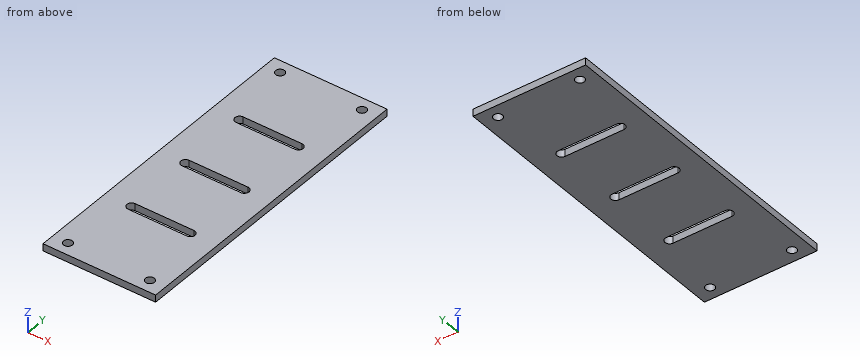
from build123d import *

# Parameters (mm, degrees)
PACK_ACCESS_WITH_STRAP_VENTILATION_PROFI_W = 44
PACK_ACCESS_WITH_STRAP_VENTILATION_PROFI_H = 120
PACK_ACCESS_WITH_STRAP_VENTILATION_PROFI_R = 1.75
PACK_ACCESS_WITH_STRAP_VENTILATION_DEPTH   = 2.8


with BuildPart() as part:
    # Pack access with strap ventilation profile → Pack access with strap ventilation (new body)
    with BuildSketch(Plane.XY):
        Rectangle(PACK_ACCESS_WITH_STRAP_VENTILATION_PROFI_W, PACK_ACCESS_WITH_STRAP_VENTILATION_PROFI_H)
        with Locations((-16, -55)):
            Circle(PACK_ACCESS_WITH_STRAP_VENTILATION_PROFI_R, mode=Mode.SUBTRACT)
        with Locations((-16, 55)):
            Circle(PACK_ACCESS_WITH_STRAP_VENTILATION_PROFI_R, mode=Mode.SUBTRACT)
        with Locations((16, -55)):
            Circle(PACK_ACCESS_WITH_STRAP_VENTILATION_PROFI_R, mode=Mode.SUBTRACT)
        with Locations((16, 55)):
            Circle(PACK_ACCESS_WITH_STRAP_VENTILATION_PROFI_R, mode=Mode.SUBTRACT)
        with BuildLine():
            Line((-11.5, -29.8), (11.5, -29.8))
            ThreePointArc((11.5, -29.8), (13.3, -28), (11.5, -26.2))
            Line((11.5, -26.2), (-11.5, -26.2))
            ThreePointArc((-11.5, -26.2), (-13.3, -28), (-11.5, -29.8))
        make_face(mode=Mode.SUBTRACT)
        with BuildLine():
            Line((-11.5, -1.8), (11.5, -1.8))
            ThreePointArc((11.5, -1.8), (13.3, 0), (11.5, 1.8))
            Line((11.5, 1.8), (-11.5, 1.8))
            ThreePointArc((-11.5, 1.8), (-13.3, 0), (-11.5, -1.8))
        make_face(mode=Mode.SUBTRACT)
        with BuildLine():
            Line((-11.5, 26.2), (11.5, 26.2))
            ThreePointArc((11.5, 26.2), (13.3, 28), (11.5, 29.8))
            Line((11.5, 29.8), (-11.5, 29.8))
            ThreePointArc((-11.5, 29.8), (-13.3, 28), (-11.5, 26.2))
        make_face(mode=Mode.SUBTRACT)
    extrude(amount=PACK_ACCESS_WITH_STRAP_VENTILATION_DEPTH)


solid = part.part
Can you work these out from the model? Positions are in its coordinate system, mm. Coordinates: 2 decimals unless noted, no trailing zeros. Order: outer loops, then holes, each group sorted by start corner. A loop starts at its lowest first (then second) coordinate and runs counter-clockwise, first axis right, second up. Notation, with made-up numbers: M 69.25,65.5 L 75.25,65.5 A5 ccw 75.25,74.5 Z; hole C 21,77 d10. An arc over 180 degrees is marked long. Answer as CSV lines item,"result".
(1) Suppose I cut it at A-A on y = 55. Please give me the cut outline in (x, z), plus the area to 3 significant figures.
Geometry check:
outline,"M -22,0 L -17.75,0 L -17.75,2.8 L -22,2.8 Z; M -14.25,0 L 14.25,0 L 14.25,2.8 L -14.25,2.8 Z; M 17.75,0 L 22,0 L 22,2.8 L 17.75,2.8 Z"
area,"104 mm^2"
(2) Suppose I cut it at D-D on x = 16. Please give me the cut outline in (y, z), plus the area to 3 significant figures.
Geometry check:
outline,"M -60,0 L -56.75,0 L -56.75,2.8 L -60,2.8 Z; M -53.25,0 L 53.25,0 L 53.25,2.8 L -53.25,2.8 Z; M 56.75,0 L 60,0 L 60,2.8 L 56.75,2.8 Z"
area,"316 mm^2"
(3) Suppose I cut it at C-C on y = -28. Please give me the cut outline in (x, z).
Geometry check:
outline,"M -22,0 L -13.3,0 L -13.3,2.8 L -22,2.8 Z; M 13.3,0 L 22,0 L 22,2.8 L 13.3,2.8 Z"
(4) Suppose I cut it at B-B on z = 0.7. Please give me the cut outline in (x, y), plus the area to 3 significant figures.
Geometry check:
outline,"M -22,-60 L 22,-60 L 22,60 L -22,60 Z; hole C -16,-55 d3.5; hole C -16,55 d3.5; hole M -11.5,-29.8 L 11.5,-29.8 A1.8 ccw 11.5,-26.2 L -11.5,-26.2 A1.8 ccw Z; hole M -11.5,-1.8 L 11.5,-1.8 A1.8 ccw 11.5,1.8 L -11.5,1.8 A1.8 ccw Z; hole M -11.5,26.2 L 11.5,26.2 A1.8 ccw 11.5,29.8 L -11.5,29.8 A1.8 ccw Z; hole C 16,-55 d3.5; hole C 16,55 d3.5"
area,"4,960 mm^2"
(5) I'm going to push a flat-ended pin straight in: pin 1 (3 mm diameter, centred on x = 16, y = -55, fed in from -Z). Where does the tip first touch, or does it pass through?
Geometry check:
pin 1,"through"
(6) Please list where these lines run through material, in increasing order: L1, parallel to Y at x = -16, z = 1.3; L2, parallel to Y at x = 6, z = 0.35; L3, parallel to Y at x = -12, z = 0.65.
Geometry check:
L1,"-60 to -56.75, -53.25 to 53.25, 56.75 to 60"
L2,"-60 to -29.8, -26.2 to -1.8, 1.8 to 26.2, 29.8 to 60"
L3,"-60 to -29.73, -26.27 to -1.73, 1.73 to 26.27, 29.73 to 60"
